Geometry check sheet. Reference: drawing and pictorial views, mm from the part's lowest x, y, z. Coordinates: 2 decimals unless noted, no trailing zeros. Loops run counter-clockwise (first coordinate to the right, second up) from the corner with the lowest first, then second, coordinate; pieces in that order, holes last. Notation, with made-up numbers: (-14, 36.5) - (8, 36.5) arc R19 cw to (8, 58.5) - close; hole circle Ø2 at (32.5, 71.5). An arc over 180 degrees is marked (long way). Write each question's results on one line, items separated by ' | '. Start each with the question number.
1. Thickness scan on line 1 (X direction, y = 15.5, z = 53); line 2 (Z direction, x = 71.5, y = 16) (1 decimal); line 3 (Z direction, x = 46, y = 15.5). Record the ranges inside material, lowest first. Write a range as [from, to].
2. Cross-section at D-D (x = 91). Record the cut outline in (y, z).
3. Gauge pin test, flat ends, axial feed: P1, Ø0.7, axis at y = 7.5, z = 51.5, coming from the +X side; P2, Ø2, axis at y = 18.5, z = 20, coming from the +X side; P3, Ø7, axis at x = 37, y = 13, coming from the -Z side (1 decimal). Record the tip position at first contact, or that the pin passes through.
4. Cross-section at C-C (z = 39). Record the cut outline in (x, y) (1 decimal).
5. Cross-section at A-A (y = 4.5). Record the cut outline in (x, z).
6. Cross-section at B-B (x = 73.5). Record the cut outline in (y, z), and give its area (3 significant figures).
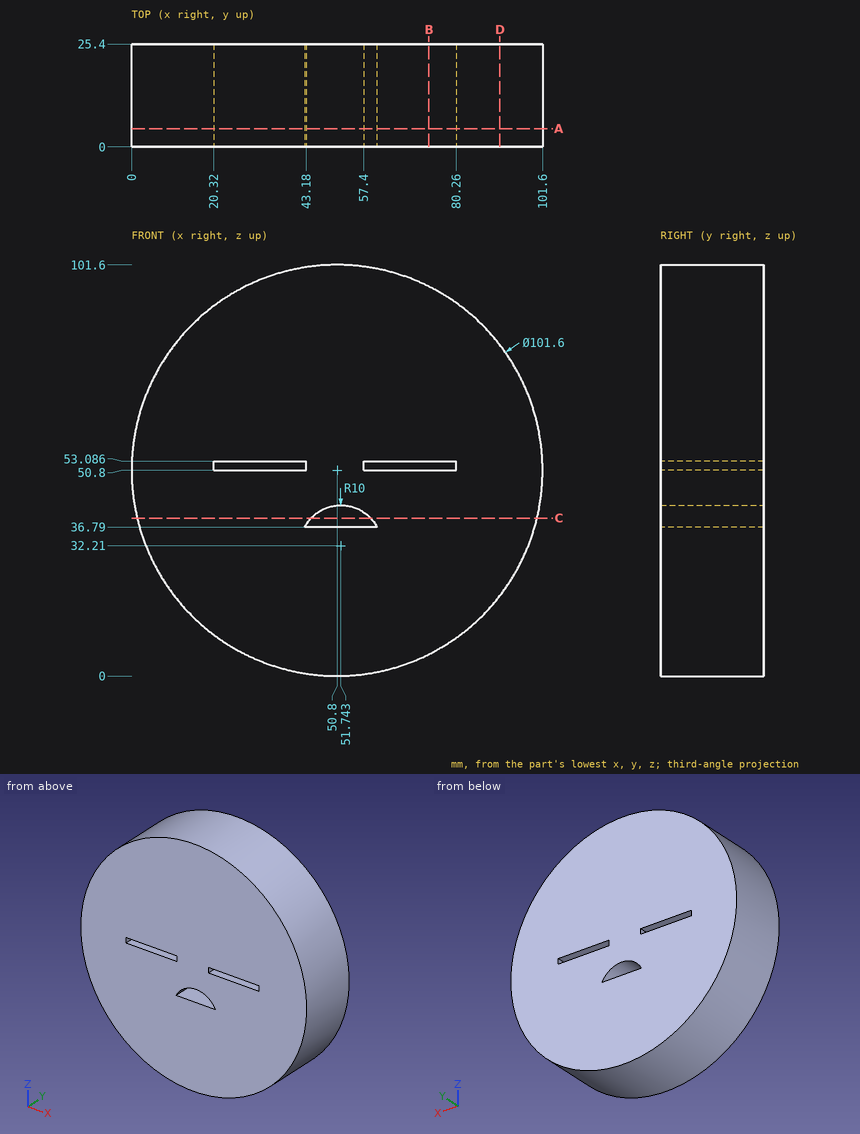
Established:
1) line 1: [0.05, 20.32], [43.18, 57.4], [80.26, 101.55] | line 2: [4.4, 50.8], [53.1, 97.2] | line 3: [0.23, 36.79], [40.4, 101.37]
2) outline: (0, 19.74) - (25.4, 19.74) - (25.4, 81.86) - (0, 81.86) - close
3) P1: x = 101.6 | P2: x = 91.94 | P3: z = 1.1
4) outline: (1.4, 0) - (44.4, 0) - (44.4, 25.4) - (1.4, 25.4) - close; (59.1, 0) - (100.2, 0) - (100.2, 25.4) - (59.1, 25.4) - close
5) outline: circle Ø101.6 at (50.8, 50.8); hole (20.32, 50.8) - (43.18, 50.8) - (43.18, 53.09) - (20.32, 53.09) - close; hole (42.85, 36.79) - (60.63, 36.79) arc R10 ccw to start; hole (57.4, 50.8) - (80.26, 50.8) - (80.26, 53.09) - (57.4, 53.09) - close
6) outline: (0, 5.35) - (25.4, 5.35) - (25.4, 50.8) - (0, 50.8) - close; (0, 53.09) - (25.4, 53.09) - (25.4, 96.25) - (0, 96.25) - close | area: 2,250 mm^2
